The model under review builds one solid part; all positions refer to its coordinate system, in mm. Face numbers are marked on the shaded views. A direction names the side the tool comes from. Coordinates: 2 decimals unless noted, no trailing zeros. Write each loop counter-clockwise with the first axis right and the second up, starting at its lowest first coordinate (ties: lowest second). Pieces come first, ordered by that corner, then holes. Notation, with made-up numbers: (2, 11) - (21, 11) arc R26 cw to (21, 41) - close; hole circle Ø9 at (35.5, -13). An arc over 180 degrees is marked (long way). Put each result on its own line as item: value. Start each with the question number.
Item 1: Consider section A-A on z = 94. Give the boundary of the cut face in (x, y).
Item 2: Consider section B-B on y = -37. Give the boundary of the cut face in (x, z).
Item 3: To check wall thickness, follow L1, parallel to X at y = -59, z = 83; L2, parallel to X at y = -50, z = 114; L3, parallel to Y at x = 0, z = 113.5. State the ranges of each line that lie inside material, in increasing order. Write a range as [from, to].
Item 4: Machinability: for the marked faces 1, 2 and 3, which of the approach directions +Z, -Z, +X, -X, +Y, -Y give a long, thin tool a straight path to every point of the face, cutting with its end or side? Answer none if there is none.
Item 5: Consider section C-C on x = -16.5. Give the boundary of the cut face in (y, z), then the cut area to 3 significant figures.
Item 6: Consider section D-D on y = -20. Give the boundary of the cut face in (x, z).
Item 7: For pin 1 (1 mm diameter, centred on y = -15.5, z = 86, fed in from -X); pin 2 (6.5 mm diameter, centred on y = -0.5, z = 41.5, fed in from +X); pin 3 (9 mm diameter, centred on y = -2, z = 21, fed in from -X), all flat-tipped, find the tip position at first contact; note any pin that passes through.
Item 8: Mouldability with a two-part tool opening along X and no side actions: class the marked faces 4, 5 and 6 as pulls with the +X half, pulls with the -X half, needs draft (parallel to the pull), parting line crosses it, or undercut.
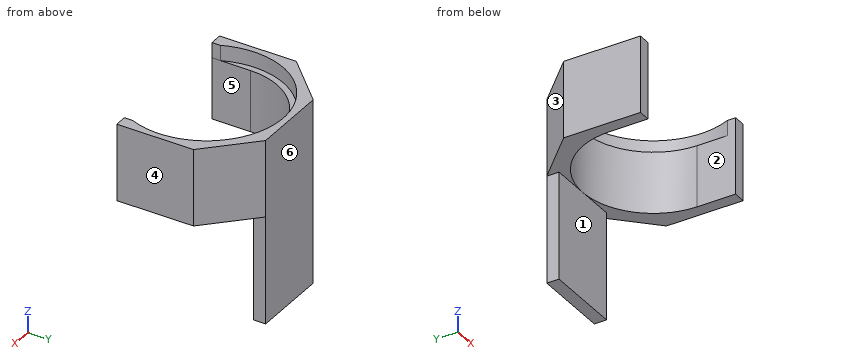
```python
from build123d import *

# Parameters (mm, degrees)
SKETCH_1_W      = 50
SKETCH_1_H      = 8
EXTRUDE_1_DEPTH = 40
EXTRUDE_2_DEPTH = 10


with BuildPart() as part:
    # 扫描1: sweep along a path in 草图2
    with BuildLine(Plane(origin=(0, 0, 0), x_dir=(0, 0, -1), z_dir=(1, 0, 0))) as sweep_1_path:
        Line((0, 55.298323556), (-110, 55.298323556))
    # 草图1 → 扫描1 (sweep)
    with BuildSketch(Plane.XY):
        Rectangle(SKETCH_1_W, SKETCH_1_H)
    sweep(path=sweep_1_path.line)

    # 草图4 → 凸台-拉伸1 (add)
    with BuildSketch(Plane.XY.offset(110)):
        with BuildLine():
            Line((-54, -25), (-25, 4))
            Line((-25, 4), (25, 4))
            Line((25, 4), (54, -25))
            Line((54, -25), (54, -75))
            Line((54, -75), (46, -75))
            Line((46, -75), (46, -50))
            ThreePointArc((46, -50), (0, -4), (-46, -50))
            Line((-46, -50), (-46, -75))
            Line((-46, -75), (-54, -75))
            Line((-54, -75), (-54, -25))
        make_face()
    extrude(amount=-EXTRUDE_1_DEPTH)

    # 草图5 → 凸台-拉伸2 (add)
    with BuildSketch(Plane.XY.offset(110)):
        with BuildLine():
            Line((-46.0046646, -69.584964515), (-46, -75))
            Line((-46, -75), (-54, -75))
            Line((-54, -75), (-54, -25))
            Line((-54, -25), (-25, 4))
            Line((-25, 4), (25, 4))
            Line((25, 4), (54, -25))
            Line((54, -25), (54, -75))
            Line((54, -75), (46, -75))
            Line((46, -75), (46, -69.595917942))
            ThreePointArc((46, -69.595917942), (0.005952648, -3.54e-07), (-46.0046646, -69.584964515))
        make_face()
    extrude(amount=EXTRUDE_2_DEPTH)


solid = part.part
```
Report:
1. outline: (-54, -75) - (-46, -75) - (-46, -50) arc R46 cw to (46, -50) - (46, -75) - (54, -75) - (54, -25) - (25, 4) - (-25, 4) - (-54, -25) - close
2. outline: (-54, 70) - (-44.12, 70) - (-44.12, 110) - (-48.28, 110) - (-48.28, 120) - (-54, 120) - close; (44.12, 70) - (54, 70) - (54, 120) - (48.28, 120) - (48.28, 110) - (44.12, 110) - close
3. L1: [-54, -46], [46, 54]
3. L2: [-54, -50], [50, 54]
3. L3: [0, 4]
4. face 1: -Z, +X, -X, -Y
4. face 2: +Z, -Z, -Y
4. face 3: +Z, -Z, -X, +Y
5. outline: (-7.06, 70) - (-4, 70) - (-4, 0) - (4, 0) - (4, 120) - (-2.8, 120) - (-2.8, 110) - (-7.06, 110) - close
5. area: 1,070 mm²
6. outline: (-49, 70) - (-34.87, 70) - (-34.87, 110) - (-40, 110) - (-40, 120) - (-49, 120) - close; (34.87, 70) - (49, 70) - (49, 120) - (40, 120) - (40, 110) - (34.87, 110) - close
7. pin 1: x = -45
7. pin 2: x = 25
7. pin 3: x = -25
8. face 4: pulls with the +X half
8. face 5: undercut
8. face 6: needs draft
